Could you check a few things on this model? Use its own coordinates, in mm. A direction names the side the tool comes from. Give positions to 0.01 mm unless a question says otherwise; leave off trailing zeros. Order: outer loops, then holes, each group sorted by start corner. A loop starts at its lowest first (then second) coordinate and runs counter-clockwise, first axis right, second up. Notation, with made-up numbers: M 3.25,-12 L 10.25,-12 A21 cw 10.25,27 Z; hole C 78.5,2.25 d6. An arc over 180 degrees is marked long. Use a Markdown table: item, result. Add a question column.
Item 1: Suppose I cut it at D-D on y = 19.75. Write out the boundary of the cut face in (x, z), plus the area to 3 significant figures.
Item 2: For faces 4 (the face through (3.711, 1.479, 11.786)), 5 (the face through (3, 3, 52)), which set-ups out of +Z, -Z, +X, -X, +Y, -Y let a thin tool reach every point of the face, with its end or its side?
Item 3: Suppose I cut it at A-A on z = 50. Write out the boundary of the cut face in (x, y).
Item 4: I'm going to push flat-ended pins straight in: pin 1 Ø1.5 at (x, z) = (8, 43) entering from -Y; pin 2 Ø3 at (x, z) = (12, 49.5) entering from +Y; pin 3 Ø2 at (x, z) = (6, 8) entering from +Y; pin 4 Ø12 at (x, y) = (21, 11) entering from +Z. Where does each tip first touch, or does it pass through?
Item 5: If I drill on L1, parallel to X at y = 1.7, z = 50; L2, parallel to Z at x = 17.75, y = 2.5; L3, parallel to Y at x = 22.5, z = 11, over which ranges is the centre line in solid material (lowest first)? Write a range as from..to.
Item 6: If we mould it in two halves opening along Z, with no side actions, what happens to faces 1 (the face through (11.96, 4.93, 57.54)), 2 (the face through (12, 6.2, 10)), 3 (the face through (17.43, 4.62, 46.91))? For each: released by +Z, released by -Z, zero draft, split by the parting line, or undercut.
Item 7: Suppose I cut it at B-B on x = 14.5. Write out the boundary of the cut face in (y, z).
Item 8: Suppose I cut it at C-C on x = 6.5. Write out the boundary of the cut face in (y, z), plus the area to 3 significant figures.
from build123d import *

# Parameters (mm, degrees)
SKETCH_1_W          = 24.26
SKETCH_1_H          = 6.2
EXTRUDE_1_DEPTH     = 60
CUT_EXTRUDE_1_DEPTH = 3.2
HOLE_WIZARD_M41_D   = 4.5
EXTRUDE_2_DEPTH     = 24.26
CHAMFER_1_SIZE      = 2.5
CHAMFER_1_SIZE2     = 5
CHAMFER_2_SIZE      = 5
CHAMFER_2_SIZE2     = 2.5


with BuildPart() as part:
    # Эскиз1 → Бобышка-Вытянуть1 (new body)
    with BuildSketch(Plane.XY):
        with Locations((12.13, 3.1)):
            Rectangle(SKETCH_1_W, SKETCH_1_H)
    extrude(amount=EXTRUDE_1_DEPTH)

    # Эскиз2 → Вырез-Вытянуть1 (cut)
    with BuildSketch(Plane(origin=(0, 6.2, 0), x_dir=(1, 0, 0), z_dir=(0, 1, 0))):
        Polygon((1.53, -47.950406544), (1.53, -52.049593456), (5.08, -54.099186911), (8.63, -52.049593456), (8.63, -47.950406544), (5.08, -45.900813089), align=None)
        Polygon((15.63, -47.950406544), (15.63, -52.049593456), (19.18, -54.099186911), (22.73, -52.049593456), (22.73, -47.950406544), (19.18, -45.900813089), align=None)
        Polygon((15.63, -7.950406544), (15.63, -12.049593456), (19.18, -14.099186911), (22.73, -12.049593456), (22.73, -7.950406544), (19.18, -5.900813089), align=None)
        Polygon((5.08, -14.099186911), (8.63, -12.049593456), (8.63, -7.950406544), (5.08, -5.900813089), (1.53, -7.950406544), (1.53, -12.049593456), align=None)
    extrude(amount=-CUT_EXTRUDE_1_DEPTH, mode=Mode.SUBTRACT)

    # Отверстие с зазором M41 (through all)
    with Locations(Plane(origin=(5.08, 3, 50), x_dir=(0, 0, 1), z_dir=(0, 1, 0))):
        with Locations((0, 0), (0, 14.1), (-40, 0), (-40, 14.1)):
            Hole(HOLE_WIZARD_M41_D / 2)

    # Эскиз6 → Бобышка-Вытянуть2 (add)
    with BuildSketch(Plane.ZY):
        with BuildLine():
            Line((40, 26.2), (20, 26.2))
            Line((20, 26.2), (20, 11.2))
            ThreePointArc((20, 11.2), (18.535533906, 7.664466094), (15, 6.2))
            Line((15, 6.2), (45, 6.2))
            ThreePointArc((45, 6.2), (41.464466094, 7.664466094), (40, 11.2))
            Line((40, 11.2), (40, 26.2))
        make_face()
    extrude(amount=-EXTRUDE_2_DEPTH)

    # Фаска1
    chamfer_1_edges = [part.edges().sort_by_distance(p)[0] for p in [
        (12.13, 6.2, 0),
    ]]
    chamfer_1_side = [part.faces().sort_by_distance(p)[0] for p in [
        (12.13, 3.1, 0),
    ]]
    chamfer(chamfer_1_edges, length=CHAMFER_1_SIZE, length2=CHAMFER_1_SIZE2, reference=chamfer_1_side[0])

    # Фаска2
    chamfer_2_edges = [part.edges().sort_by_distance(p)[0] for p in [
        (12.13, 6.2, 60),
    ]]
    chamfer_2_side = [part.faces().sort_by_distance(p)[0] for p in [
        (12.13, 6.2, 53.289196352),
    ]]
    chamfer(chamfer_2_edges, length=CHAMFER_2_SIZE, length2=CHAMFER_2_SIZE2, reference=chamfer_2_side[0])


solid = part.part
Findings below:
| question | item | result |
|---|---|---|
| 1 | outline | M 0,20 L 24.26,20 L 24.26,40 L 0,40 Z |
| 1 | area | 485 mm^2 |
| 2 | face 4 | +Y, -Y |
| 2 | face 5 | +Y |
| 3 | outline | M 0,0 L 2.83,0 L 2.83,3 L 1.53,3 L 1.53,6.2 L 0,6.2 Z; M 7.33,0 L 16.93,0 L 16.93,3 L 15.63,3 L 15.63,6.2 L 8.63,6.2 L 8.63,3 L 7.33,3 Z; M 21.43,0 L 24.26,0 L 24.26,6.2 L 22.73,6.2 L 22.73,3 L 21.43,3 Z |
| 4 | pin 1 | stops at y = 0 |
| 4 | pin 2 | stops at y = 6.2 |
| 4 | pin 3 | stops at y = 3 |
| 4 | pin 4 | stops at z = 57.4 |
| 5 | L1 | x = 0..2.83, 7.33..16.93, 21.43..24.26 |
| 5 | L2 | z = 0..8.26, 11.74..48.26, 51.74..60 |
| 5 | L3 | y = 0..3 |
| 6 | face 1 | released by +Z |
| 6 | face 2 | zero draft |
| 6 | face 3 | undercut |
| 7 | outline | M 0,0 L 3.7,0 L 6.2,5 L 6.2,15 A5 cw 11.2,20 L 26.2,20 L 26.2,40 L 11.2,40 A5 cw 6.2,45 L 6.2,55 L 3.7,60 L 0,60 Z |
| 8 | outline | M 0,0 L 3.7,0 L 6.2,5 L 6.2,6.72 L 3,6.72 L 3,8.25 L 0,8.25 Z; M 0,11.75 L 3,11.75 L 3,13.28 L 6.2,13.28 L 6.2,15 A5 cw 11.2,20 L 26.2,20 L 26.2,40 L 11.2,40 A5 cw 6.2,45 L 6.2,46.72 L 3,46.72 L 3,48.25 L 0,48.25 Z; M 0,51.75 L 3,51.75 L 3,53.28 L 6.2,53.28 L 6.2,55 L 3.7,60 L 0,60 Z |
| 8 | area | 707 mm^2 |
